from build123d import *

# Parameters (mm, degrees)
F2_SIZE = 0.5
F3_SIZE = 1


with BuildPart() as f1:
    # F0 (on Top) → F1 (revolve)
    with BuildSketch(Plane.XY):
        with BuildLine():
            Line((-34.5, 25.4), (-34.5, 22.75))
            Line((-34.5, 22.75), (-25.8, 22.75))
            Line((-25.8, 22.75), (-23, 22.75))
            add(Edge.make_bspline(
                [(-23, 22.75), (-22.4767401814, 23.4261993319), (-21.5331446379, 23.6), (-20, 23.6)],
                knots=[0, 0, 0, 0, 3.1180923655, 3.1180923655, 3.1180923655, 3.1180923655], degree=3))
            Line((-20, 23.6), (0, 23.6))
            Line((0, 23.6), (0, 24.55))
            Line((0, 24.55), (-25.8, 24.55))
            add(Edge.make_bspline(
                [(-28.8, 25.4), (-28.3960923553, 25.0019170344), (-27.5980718434, 24.6472395957), (-25.8, 24.55)],
                knots=[0, 0, 0, 0, 3.1180923655, 3.1180923655, 3.1180923655, 3.1180923655], degree=3))
            Line((-28.8, 25.4), (-34.5, 25.4))
        make_face()
    revolve(axis=Axis((-33.9306145906, 0, 0), (-1, 0, 0)))

    # F2
    f2_edges = [f1.edges().sort_by_distance(p)[0] for p in [
        (-34.5, -25.4, 0),
    ]]
    chamfer(f2_edges, length=F2_SIZE)

    # F3
    f3_edges = [f1.edges().sort_by_distance(p)[0] for p in [
        (-34.5, -22.75, 0),
    ]]
    chamfer(f3_edges, length=F3_SIZE)

    # F4: F1 across face


with BuildPart() as f1_1:
    add(f1.part)
    add(f1.part.mirror(Plane.YZ))


solid = f1_1.part
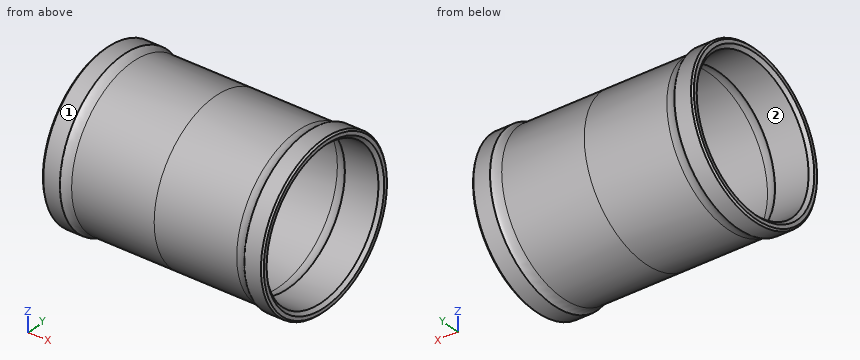
Geometry: final body of the model. Coordinates: model frame, mm. Face numbers are marked on the shaded views. Give positions to 0.01 mm unless a question says otherwise; leave off trailing zeros. Loops run counter-clockwise (first coordinate to the right, second up) from the corner with the lowest first, then second, coordinate; pieces in that order, holes last. Notation, with made-up numbers: (-2.75, 33.25) -> (24.25, 33.25) arc R30 ccw to (24.25, 55.25) -> close; hole circle Ø5 at (-29, 21.5). An arc over 180 degrees is marked (long way). Put each result on its own line as item: value.
1. Pull-direction query (Z, two-part tool) for the marked faces 1 and 2; classes: released by +Z, released by -Z, zero draft, split by the parting line, or undercut.
Taken from the geometry:
face 1: split by the parting line
face 2: undercut
2. Pin query (flat end, axial travel): P1, Ø3, axis at x = -3.5, z = -6, coming from the +Y side; P2, Ø8, axis at y = -18.5, z = -6, coming from the +X side; P3, Ø10, axis at x = -4.5, y = -6.5, coming from the +Z side. Return the tip coordinate at first contact, or that it passes through.
Taken from the geometry:
P1: stops at y = 24.13
P2: stops at x = 34.2
P3: stops at z = 24.5
3. Ray query, line 1 along Z through (x, y) = (-30.75, 0); line 2 along Z through (x, y) = (-26, 0); line 3 along Y through (x, z) = (-25.5, 0). Return the intervals inside material, ascending. Write a range as [from, to].
Taken from the geometry:
line 1: z = [-25.4, -22.75], [22.75, 25.4]
line 2: z = [-24.56, -22.75], [22.75, 24.56]
line 3: y = [-24.55, -22.75], [22.75, 24.55]
4. Cut plane A-A (x = -17.5). Return the cut outline in (y, z).
Taken from the geometry:
outline: circle Ø49.1 at (0, 0); hole circle Ø47.2 at (0, 0)
